from build123d import *

# Parameters (mm, degrees)
F0_R     = 32.5
F1_DEPTH = 10
F2_R     = 12.5
F3_DEPTH = 10
F4_R     = 10
F5_DEPTH = 20
F6_R     = 30
F6_R_2   = 29.5
F7_DEPTH = 3


with BuildPart() as f1:
    # F0 (on Front) → F1 (new body)
    with BuildSketch(Plane.XZ):
        Circle(F0_R)
    extrude(amount=-F1_DEPTH)

    # F2 (on face) → F3 (join)
    with BuildSketch(Plane.XZ):
        Circle(F2_R)
    extrude(amount=F3_DEPTH)

    # F4 (on face) → F5 (cut)
    with BuildSketch(Plane.XZ.offset(10)):
        Circle(F4_R)
    extrude(amount=-F5_DEPTH, mode=Mode.SUBTRACT)

    # F6 (on face) → F7 (join)
    with BuildSketch(Plane(origin=(0, 10, 0), x_dir=(-1, 0, 0), z_dir=(0, 1, 0))):
        Circle(F6_R)
        Circle(F6_R_2, mode=Mode.SUBTRACT)
    extrude(amount=F7_DEPTH)


solid = f1.part
Here's how the part is built. I have some questions about the finished solid (model axes, mm). A direction names the side the tool comes from. Give positions to 0.01 mm unless a question says otherwise; leave off trailing zeros. Loops run counter-clockwise (first coordinate to the right, second up) from the corner with the lowest first, then second, coordinate; pieces in that order, holes last. Notation, with made-up numbers: (75, -40) -> (131, -40) arc R19 cw to (131, -12) -> close; hole circle Ø6 at (67, 32). An arc over 180 degrees is marked (long way). One line per item, written item: value.
Q1. Suppose I cut it at C-C on y = 8.5. Please give me the cut outline in (x, z), then the cut area to 3 significant figures.
Answers follow:
outline: circle Ø65 at (0, 0); hole circle Ø20 at (0, 0)
area: 3,000 mm^2
Q2. Suppose I cut it at D-D on z = -16.5. Please give me the cut outline in (x, y), then the cut area to 3 significant figures.
Answers follow:
outline: (-28, 0) -> (28, 0) -> (28, 10) -> (25.05, 10) -> (25.05, 13) -> (24.45, 13) -> (24.45, 10) -> (-24.45, 10) -> (-24.45, 13) -> (-25.05, 13) -> (-25.05, 10) -> (-28, 10) -> close
area: 564 mm^2
Q3. On a 3-axis mill with a long thin cutter (end or side, diameter ignored), from which of +Z, -Z, +X, -X, +Y, -Y can I reach the whole of each face in a straight line? I mean faces 1 (the face through (-0.1, -10, 10.2)), 2 (the face through (-28.14, 11.48, 8.86)), 3 (the face through (11.923, -4.93, 3.755)). Say none if no direction works.
Answers follow:
face 1: +Z, -Z, +X, -X, -Y
face 2: +Y
face 3: -Y
Q4. We'd pull the mould along Z, two halves only. Please class faces 4 (the face through (31, 4.93, 9.76)), 5 (the face through (9, 10, -29)), 6 (the face through (13, 10, 0)): pulls with the +Z half, pulls with the -Z half, needs draft (parallel to the pull), parting line crosses it, or undercut.
Answers follow:
face 4: parting line crosses it
face 5: needs draft
face 6: undercut
Q5. Suppose I cut it at B-B on x = 0. Please give me the cut outline in (y, z).
Answers follow:
outline: (-10, -12.5) -> (0, -12.5) -> (0, -32.5) -> (10, -32.5) -> (10, -30) -> (13, -30) -> (13, -29.5) -> (10, -29.5) -> (10, -10) -> (-10, -10) -> close; (-10, 10) -> (10, 10) -> (10, 29.5) -> (13, 29.5) -> (13, 30) -> (10, 30) -> (10, 32.5) -> (0, 32.5) -> (0, 12.5) -> (-10, 12.5) -> close
Q6. If I drill on line 1 along Z through (x, y) = (0, 4); line 2 along Z through (x, y) = (0, 12.35); line 3 along Y through (x, z) = (-1.5, -25.5), over which ranges is the centre line in solid material (lowest first)?
Answers follow:
line 1: -32.5 to -10, 10 to 32.5
line 2: -30 to -29.5, 29.5 to 30
line 3: 0 to 10
Q7. I'm going to push flat-ended pins straight in: pin 1 Ø10 at (y, z) = (9.5, 6.5) entering from +X; pin 2 Ø6 at (x, z) = (-8, -25) entering from -Y; pin 3 Ø1 at (y, z) = (9, -11.5) entering from +X. Where does each tip first touch, or does it pass through?
Answers follow:
pin 1: x = 32.47
pin 2: y = 0
pin 3: x = 30.58
Q8. Suppose I cut it at A-A on z = 0. Please give me the cut outline in (x, y), then the cut area to 3 significant figures.
Answers follow:
outline: (-32.5, 0) -> (-12.5, 0) -> (-12.5, -10) -> (-10, -10) -> (-10, 10) -> (-29.5, 10) -> (-29.5, 13) -> (-30, 13) -> (-30, 10) -> (-32.5, 10) -> close; (10, -10) -> (12.5, -10) -> (12.5, 0) -> (32.5, 0) -> (32.5, 10) -> (30, 10) -> (30, 13) -> (29.5, 13) -> (29.5, 10) -> (10, 10) -> close
area: 503 mm^2
